Study the drawing (mm; zero at the part's minimum x, y, z) and answer. Coordinates: 2 decimals unless noted, no trailing zeros. Loops run counter-clockwise (first coordinate to the right, second up) from the corner with the lowest first, then second, coordinate; pieces in that order, holes last.
Q1. Flat-ended cylindrical pins translate along their axes: P1, Ø0.8, axis at x = 3, z = 0.5, coming from the -Y side; P2, Ø0.8, axis at x = 9, z = 1, coming from the +Y side; P3, Ø6, axis at x = 23, y = 18, coming from the -Z side; P4, Ø0.8, axis at x = 21.5, z = 0.5, coming from the -Y side. Find the tip coordinate at first contact, or state that the pin passes through.
Q2. Section B-B (x = 29.25) is taken. Give the vertices of the cut face in (y, z).
Q3. Section D-D (x = 23) is taken. Give the vertices of the cut face in (y, z).
Q4. Section A-A (y = 21.25) is taken. Give the vertices of the cut face in (x, z), then the cut area to 3 significant figures.
Q5. Straight lines are drawn through the part: line 1 (X direction, y = 9.25, z = 1.4); line 2 (Y direction, x = 23.5, z = 1.25); line 3 (Y direction, x = 7, z = 1.25). For each, find the intervals that lie inside material, in ascending order.
Q6. Section C-C (z = 0.6) is taken. Give the vertices of the cut face in (x, y).
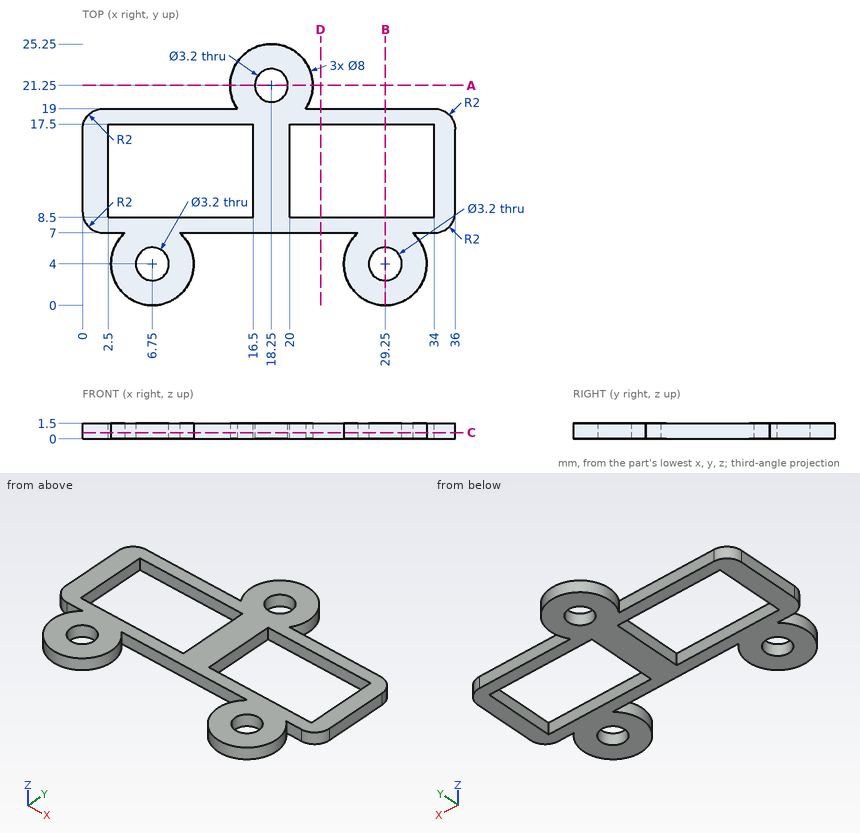
Numbers:
1. P1: stops at y = 1.81
1. P2: stops at y = 19
1. P3: stops at z = 0
1. P4: stops at y = 7
2. outline: (0, 0) - (2.4, 0) - (2.4, 1.5) - (0, 1.5) - close; (5.6, 0) - (8.5, 0) - (8.5, 1.5) - (5.6, 1.5) - close; (17.5, 0) - (19, 0) - (19, 1.5) - (17.5, 1.5) - close
3. outline: (7, 0) - (8.5, 0) - (8.5, 1.5) - (7, 1.5) - close; (17.5, 0) - (19, 0) - (19, 1.5) - (17.5, 1.5) - close
4. outline: (14.25, 0) - (16.65, 0) - (16.65, 1.5) - (14.25, 1.5) - close; (19.85, 0) - (22.25, 0) - (22.25, 1.5) - (19.85, 1.5) - close
4. area: 7.20 mm2
5. line 1: x = 0 to 2.5, 16.5 to 20, 34 to 36
5. line 2: y = 7 to 8.5, 17.5 to 19
5. line 3: y = 0.01 to 2.42, 5.58 to 8.5, 17.5 to 19
6. outline: (0, 9) arc R2 ccw to (2, 7) - (4.1, 7) arc R4 ccw (long way) to (9.4, 7) - (26.6, 7) arc R4 ccw (long way) to (31.9, 7) - (34, 7) arc R2 ccw to (36, 9) - (36, 17) arc R2 ccw to (34, 19) - (21.56, 19) arc R4 ccw (long way) to (14.94, 19) - (2, 19) arc R2 ccw to (0, 17) - close; hole (2.5, 8.5) - (16.5, 8.5) - (16.5, 17.5) - (2.5, 17.5) - close; hole circle Ø3.2 at (6.75, 4); hole circle Ø3.2 at (18.25, 21.25); hole (20, 8.5) - (34, 8.5) - (34, 17.5) - (20, 17.5) - close; hole circle Ø3.2 at (29.25, 4)
